Source: CAD feature listing. Evaluate the final solid. Frame: model axes, mm. Face numbers are marked on the shaded views. A direction names the side the tool comes from. Give positions to 0.01 mm unless a question says otherwise; leave off trailing zeros. Order: outer loops, then holes, each group sorted by start corner. A loop starts at its lowest first (then second) coordinate and runs counter-clockwise, first axis right, second up. Notation, with made-up numbers: (-25.75, -19) - (18.25, -19) arc R13 cw to (18.25, 1) - close; hole circle Ø6 at (82.25, 26.25). An arc over 180 degrees is marked (long way). One line per item, written item: value. Start each with the question number.
from build123d import *

# Parameters (mm, degrees)
SKETCH1_W                = 69.85
SKETCH1_H                = 76.2
SKETCH1_W_2              = 3.175
SKETCH1_H_2              = 50.8
BOSS_EXTRUDE1_DEPTH      = 6.35
BOSS_EXTRUDE2_DEPTH      = 43.18
BOSS_EXTRUDE2_DEPTH_BACK = 6.35
SKETCH1_3_W              = 3.175
SKETCH1_3_H              = 50.8
CHAMFER1_SIZE            = 12.7


with BuildPart() as part:
    # Sketch1 → Boss-Extrude1 (new, symmetric)
    # profile 1 of 3: a face of its own
    with BuildSketch(Plane(origin=(0, 0, 0), x_dir=(1, 0, 0), z_dir=(0, 1, 0))):
        Rectangle(SKETCH1_W, SKETCH1_H)
        Rectangle(SKETCH1_W_2, SKETCH1_H_2, mode=Mode.SUBTRACT)
    # profile 2 of 3: a face of its own
    with BuildSketch(Plane(origin=(0, 0, 0), x_dir=(1, 0, 0), z_dir=(0, 1, 0))):
        with BuildLine():
            Line((-34.925, 38.1), (34.925, 38.1))
            ThreePointArc((34.925, 38.1), (0, 51.685255393), (-34.925, 38.1))
        make_face()
    # profile 3 of 3: a face of its own
    with BuildSketch(Plane(origin=(0, 0, 0), x_dir=(1, 0, 0), z_dir=(0, 1, 0))):
        with BuildLine():
            ThreePointArc((-34.925, -38.1), (0, -51.685255393), (34.925, -38.1))
            Line((34.925, -38.1), (-34.925, -38.1))
        make_face()
    extrude(amount=BOSS_EXTRUDE1_DEPTH, both=True)

    # Sketch1<3> → Boss-Extrude2 (add, two sides: drawn at the far end of the back side and taken through both)
    with BuildSketch(Plane(origin=(0, 0, 0), x_dir=(1, 0, 0), z_dir=(0, 1, 0)).offset(-BOSS_EXTRUDE2_DEPTH_BACK)):
        Rectangle(SKETCH1_3_W, SKETCH1_3_H)
    extrude(amount=BOSS_EXTRUDE2_DEPTH + BOSS_EXTRUDE2_DEPTH_BACK)

    # Chamfer1
    chamfer1_edges = [part.edges().sort_by_distance(p)[0] for p in [
        (0, 43.18, -25.4),
    ]]
    chamfer(chamfer1_edges, length=CHAMFER1_SIZE)


solid = part.part
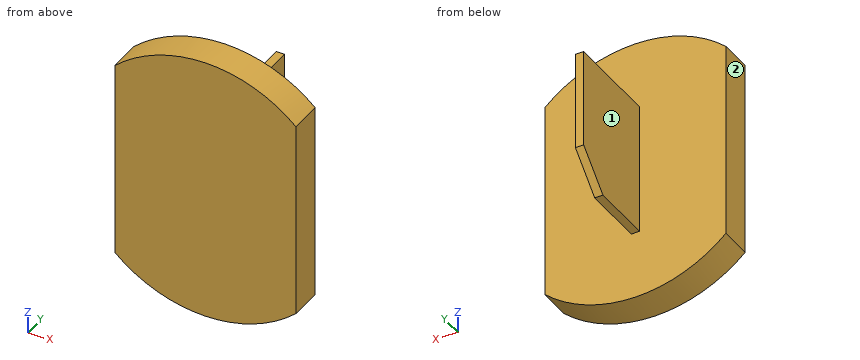
1. Section C-C on x = -14. Return the cut outline in (y, z).
2. Section B-B on y = 14. Return the cut outline in (x, z).
3. Contact query for flat-ended pins moving along their axis: pin 1 Ø1 at (x, y) = (0.5, 20) entering from -Z; pin 2 Ø5 at (x, y) = (12, 1.5) entering from -Z; pin 3 Ø1.5 at (x, z) = (11.5, 37.5) entering from +Y. Output: stop coordinate, or through.
4. Set-up query: the marked faces 1 and 2. Return all of +Z, -Z, +X, -X, +Y, -Y with unobstructed straight access to the full face (end or side cutting, diameter ignored); none if empty.
5. Ray query, L1, parallel to Y at x = -20, z = -37; L2, parallel to Z at x = -0.5, y = 11. Return the intervals inside material, ascending.
Data:
1. outline: (-6.35, -49.75) - (6.35, -49.75) - (6.35, 49.75) - (-6.35, 49.75) - close
2. outline: (-1.59, -25.4) - (1.59, -25.4) - (1.59, 25.4) - (-1.59, 25.4) - close
3. pin 1: stops at z = -25.4
3. pin 2: stops at z = -50.8
3. pin 3: stops at y = 6.35
4. face 1: +Z, -Z, -X, +Y
4. face 2: +Z, -Z, -X, +Y, -Y
5. L1: y = -6.35 to 6.35
5. L2: z = -25.4 to 25.4
